Autodesk Inventor part; units mm, degrees
ref_plane "YZ Plane" through (0, 0, 0) normal (1, 0, 0) x (0, 1, 0)
ref_plane "XZ Plane" through (0, 0, 0) normal (0, 1, 0) x (-1, 0, 0)
ref_plane "XY Plane" through (0, 0, 0) normal (0, 0, 1) x (1, 0, 0)
sketch "Sketch1" plane through (0, 0, 0) normal (0, 1, 0) x (-1, 0, 0)
  line L0 (0, 0) -> (40, 0)
  line L1 (40, 0) -> (0, -40)
  line L2 (0, -40) -> (0, 0)
  dimension "d0" = 40
  dimension "d1" = 40
extrude "Extrusion1" add sketch "Sketch1" along normal blind 9
sketch "Sketch2" plane through (0, 9, 0) normal (0, 1, 0) x (1, 0, 0)
  line L0 (-37, 3) -> (-3, 3)
  line L1 (-3, 3) -> (-3, 37)
  line L2 (-3, 37) -> (-37, 3)
  line L3 (0, 0) -> (0, 40)
  line L4 (-40, 0) -> (0, 0)
  line L5 (0, 40) -> (-40, 0)
  dimension "d4" = 3
  dimension "d5" = 3
extrude "Extrusion2" cut sketch "Sketch2" against normal blind 7 contours L2 L1 L0
sketch "Sketch3" plane through (0, 2, 0) normal (0, 1, 0) x (1, 0, 0)
  line L0 (-24.9289, 8) -> (-11.5363, 8)
  line L1 (-11.5363, 8) -> (-18.2326, 14.6963)
  line L2 (-18.2326, 14.6963) -> (-24.9289, 8)
  line L3 (-37, 3) -> (-3, 37)
  line L4 (-3, 3) -> (-37, 3)
  line L5 (-8, 11.5357) -> (-8, 24.9289)
  line L6 (-8, 24.9289) -> (-14.6966, 18.2323)
  line L7 (-14.6966, 18.2323) -> (-8, 11.5357)
  line L8 (-3, 37) -> (-3, 3)
  line L9 (-40, 0) -> (0, 0)
  line L10 (0, 0) -> (0, 40)
  dimension "d8" = 5
  dimension "d9" = 5
  dimension "d10" = 5
  dimension "d11" = 5
  dimension "d12" = 45
  dimension "d13" = 45
  dimension "d14" = 21.5415
  dimension "d16" = 9.47
extrude "Extrusion3" cut sketch "Sketch3" against normal through all contours L2 L1 L0 | L7 L6 L5
sketch "Sketch4" plane through (0, 0, 0) normal (1, 0, 0) x (0, 0, -1)
  circle A0 centre (10, 5.5) radius 1.75
  circle A1 centre (20, 5.5) radius 1.75
  line L0 (0, 0) -> (40, 0)
  circle A2 centre (30, 5.5) radius 1.75
  line L1 (0, 0) -> (0, 9)
  line L2 (40, 0) -> (40, 9)
  dimension "d19" = 3.5
  dimension "d20" = 3.5
  dimension "d21" = 5.5
  dimension "d22" = 5.5
  dimension "d23" = 3.5
  dimension "d24" = 5.5
  dimension "d25" = 20
  dimension "d26" = 10
  dimension "d27" = 10
sketch "Sketch5" plane through (-40, 0, 0) normal (0, 0, 1) x (1, 0, 0)
  circle A0 centre (10, 5.5) radius 1.75
  circle A1 centre (20, 5.5) radius 1.75
  circle A2 centre (30, 5.5) radius 1.75
  line L0 (0, 0) -> (40, 0)
  line L1 (40, 0) -> (40, 9)
  line L2 (0, 0) -> (0, 9)
  dimension "d30" = 3.5
  dimension "d31" = 3.5
  dimension "d32" = 3.5
  dimension "d33" = 5.5
  dimension "d34" = 5.5
  dimension "d35" = 10
  dimension "d36" = 5.5
  dimension "d37" = 20
  dimension "d38" = 10
extrude "Extrusion6" cut sketch "Sketch4" against normal through all
extrude "Extrusion7" cut sketch "Sketch5" against normal through all
fillet "Fillet1" radius 1 2 edges at (0, 4.5, -40) (-40, 4.5, 0)
chamfer "Chamfer1" distance 1.5 angle 45 8 edges at (-21.5808, 2, -11.3482) (-18.2326, 2, -8) (-14.8845, 2, -11.3482) (-11.3483, 2, -14.884) (-11.3483, 2, -21.5806) (-8, 2, -18.2323) (-20, 9, -3) (-3, 9, -20)
chamfer "Chamfer2" distance 1 angle 45 6 edges at (-31.75, 5.5, -3) (-21.75, 5.5, -3) (-11.75, 5.5, -3) (-3, 5.5, -8.25) (-3, 5.5, -18.25) (-3, 5.5, -28.25)
properties part number "equerre_droite"
Could you check a few things on this model? Use its own coordinates, in mm. A direction names the side the tool comes from. Give positions to 0.01 mm unless a question says otherwise; leave off trailing zeros. Write each loop counter-clockwise with the first axis right and the second up, starting at its lowest first coordinate (ties: lowest second). Pieces come first, ordered by that corner, then holes. Notation, with made-up numbers: (-21, 10) -> (-10, 10) arc R23 ccw to (-10, 42) -> close; hole circle Ø9 at (-36, 48). An arc over 180 degrees is marked (long way). Answer as CSV lines item,"result". Start each with the question number.
(1) If we section it at C-C, the plane z = -30: Write out the boundary of the cut face in (x, y) (3 decimals), and give its area (3 significant figures).
(2) Which directions (+Z, -Z, +X, -X, +Y, -Y) give clear straight access to the entire face, cutting with the end or side of a thin tool? Please do faces 1 (the face through (-2.3, 8.2, -20.2)), 2 (the face through (-21.53, 0.25, -11.4)), 3 (the face through (-0.602, 4.563, -38.503)).
(3) Please list where these lines run through material, in increasing order: line 1 (Y direction, x = -20, z = -1); line 2 (X direction, y = 3.25, z = -27); line 3 (Z direction, x = -22.5, y = 1.25).
(4) If we section it at B-B, the plane x = -20: Write out the boundary of the cut face in (y, z) (3 decimals), and give its area (3 significant figures).
(5) If we section it at A-A, the plane z = -3.5: Write out the boundary of the cut face in (x, y).
(6) If we mould it in two halves opening along X, with no side actions, what happens to faces 4 (the face through (-2.174, 3.593, -29.75)), 5 (the face through (-19, 3, 0)), 6 (the face through (-11.3, 0.25, -21.63)), 7 (the face through (-30.25, 3.593, -2.174))? For each: +X half, -X half, draft (parallel to the pull), parting line (faces both ways), or undercut.
(7) I'm going to push flat-ended pins straight in: pin 1 Ø4.5 at (x, y) = (-10, 5.5) entering from +Z; pin 2 Ø6 at (x, z) = (-27.5, -8) entering from +Y; pin 3 Ø3 at (x, y) = (-30, 5.5) entering from -Z; pin 4 Ø1.6 at (x, y) = (-27, 3.5) entering from -Z. Where does each tip first touch, or does it pass through?
(8) If we section it at D-D, the plane x = -4: Write out the boundary of the cut face in (y, z), and give its area (3 significant figures).
Answer list:
1,outline,"(-10, 0) -> (0, 0) -> (0, 3.75) -> (-2, 3.75) -> (-3, 2.75) -> (-3, 2) -> (-10, 2) -> close; (-2.625, 7.875) -> (-2, 7.25) -> (0, 7.25) -> (0, 9) -> (-1.5, 9) -> close"
1,area,"28.5 mm^2"
2,face 1,"-Z, -X, +Y"
2,face 2,"+Y, -Y"
2,face 3,"-Z, +Y, -Y"
3,line 1,"0 to 3.75, 7.25 to 9"
3,line 2,"-3 to 0"
3,line 3,"-17.5 to -11.49, -7.25 to 0"
4,outline,"(0, -20) -> (2, -20) -> (2, -15.05) -> (0.5, -12.929) -> (0, -12.929) -> close; (0, -8) -> (0.5, -8) -> (2, -6.5) -> (2, -3) -> (2.75, -3) -> (3.75, -2) -> (3.75, 0) -> (0, 0) -> close; (7.25, -2) -> (7.875, -2.625) -> (9, -1.5) -> (9, 0) -> (7.25, 0) -> close"
4,area,"35.9 mm^2"
5,outline,"(-36.5, 0) -> (0, 0) -> (0, 9) -> (-1.5, 9) -> (-3, 7.5) -> (-3, 2) -> (-36.5, 2) -> close"
6,face 4,"-X half"
6,face 5,"draft"
6,face 6,"undercut"
6,face 7,"undercut"
7,pin 1,"z = 0"
7,pin 2,"y = 2"
7,pin 3,"through"
7,pin 4,"z = -3"
8,outline,"(0, -36) -> (2, -36) -> (2, -3) -> (7.5, -3) -> (9, -1.5) -> (9, 0) -> (0, 0) -> close"
8,area,"91.9 mm^2"
